Can you work these out from the model? Positions are in its coordinate system, mm. Give positions to 0.01 mm unless a question says otherwise; leave off trailing zeros. Order: outer loops, then holes, each group sorted by start corner. A loop starts at its lowest first (then second) coordinate and runs counter-clockwise, first axis right, second up. Notation, with made-up numbers: M -10.75,-29 L 42.25,-29 A19 cw 42.25,-25 Z; hole C 40.25,25.5 d2. An arc over 180 degrees is marked long. One line per question, with ' | ' between items. Start each with the question number.
1) If we section it at A-A, the plane y = 2.5: Please give me the cut outline in (x, z) (1 decimal).
2) I'm going to push flat-ended pins straight in: pin 1 Ø1.1 at (x, z) = (-29, 2) entering from +Y; pin 2 Ø8 at (x, z) = (-2, -164.5) entering from -Y. Where does each tip first touch, or does it pass through?
3) If we section it at B-B, the plane z = -77.5: Please give me the cut outline in (x, y).
4) Please list where these lines run through material, in increasing order: line 1 along Z through (x, y) = (-21, 2.55) (1 decimal); line 2 along X through (y, z) = (0.9, -141); line 3 along Z through (x, y) = (-38.5, 1.1) (1 decimal). Write a range as [from, to].
Autodesk Inventor part; units mm, degrees
ref_plane "YZ Plane" through (0, 0, 0) normal (1, 0, 0) x (0, 1, 0)
ref_plane "XZ Plane" through (0, 0, 0) normal (0, 1, 0) x (-1, 0, 0)
ref_plane "XY Plane" through (0, 0, 0) normal (0, 0, 1) x (1, 0, 0)
sketch "Sketch1" plane through (0, 0, 0) normal (0, 1, 0) x (-1, 0, 0)
  line L0 (0, 0) -> (50, 0)
  line L1 (50, 0) -> (50, -447.675)
  line L2 (50, -447.675) -> (0, -447.675)
  line L3 (0, -447.675) -> (0, 0)
  dimension "d0" = 50
  dimension "d1" = 447.675
extrude "Extrusion1" add sketch "Sketch1" along normal blind 4.7625
sketch "Sketch2" plane through (-50, 0, 0) normal (0, 0, 1) x (1, 0, 0)
  line L0 (1.1907, 3.5648) -> (1.1907, 1.1907)
  line L1 (50, 0) -> (0, 0)
  line L2 (50, 4.7625) -> (0, 4.7625)
  line L3 (1.1907, 1.1907) -> (48.8093, 1.1907)
  line L4 (1.1907, 3.5648) -> (48.8093, 3.5648)
  line L5 (48.8093, 3.5648) -> (48.8093, 1.1907)
  line L6 (50, 0) -> (50, 4.7625)
extrude "Extrusion2" add sketch "Sketch2" along normal blind 4.7625
sketch "Sketch3" plane through (0, 4.7625, 0) normal (0, 1, 0) x (1, 0, 0)
  line L0 (-50, 447.675) -> (-50, 0)
  line L1 (-50, 447.675) -> (-25, 447.675)
  line L2 (0, 447.675) -> (-50, 447.675)
  line L3 (-25, 447.675) -> (-25, 382.675)
  line L4 (-31, 382.675) -> (-19, 382.675)
  line L5 (-31, 382.675) -> (-31, 0)
  line L6 (-1.1907, 0) -> (-48.8093, 0)
  line L7 (-19, 382.675) -> (-19, 0)
  line L8 (-31, 0) -> (-19, 0)
  point P0 (0, 0)
  dimension "d11" = 25
extrude "Extrusion3" cut sketch "Sketch3" against normal blind 10
sketch "Sketch4" plane through (-50, 0, 4.7625) normal (0, 0, 1) x (1, 0, 0)
  line L0 (31, 3.5648) -> (31, 1.1907)
  line L1 (31, 1.1907) -> (31, 3.5648)
  line L2 (19, 3.5648) -> (31, 3.5648)
  line L3 (31, 3.5648) -> (19, 3.5648)
  line L4 (19, 3.5648) -> (19, 1.1907)
  line L5 (19, 1.1907) -> (31, 1.1907)
  point P0 (50, 0)
extrude "Extrusion4" cut sketch "Sketch4" against normal blind 10
sketch "Sketch5" plane through (0, 4.7625, 0) normal (0, 1, 0) x (1, 0, 0)
  point P0 (0, 0)
sketch "Sketch6" plane through (-31, 4.7625, -382.675) normal (0, 0, 1) x (1, 0, 0)
  line L0 (12, -4.7625) -> (0, -4.7625)
  line L1 (12, 0) -> (12, -4.7625)
  line L2 (0, 0) -> (12, 0)
  line L3 (0, 0) -> (0, -4.7625)
  point P0 (31, -4.7625)
extrude "Extrusion5" add sketch "Sketch6" along normal blind 158.838
sketch "Sketch8" plane through (-31, 4.7625, -223.837) normal (0, 0, 1) x (1, 0, 0)
  line L0 (3.6185, -4.7625) -> (3.6185, 0)
  line L1 (3.6185, 0) -> (8.3815, 0)
  line L2 (8.3815, 0) -> (8.3815, -4.7625)
  line L3 (3.6185, -4.7625) -> (8.3815, -4.7625)
  line L4 (0, -4.7625) -> (12, -4.7625)
  line L5 (-19, 0) -> (0, 0)
  line L6 (0, 0) -> (3.6185, 0)
  line L7 (12, 0) -> (0, 0)
  line L8 (3.6185, -4.7625) -> (0, -4.7625)
  line L9 (0, -4.7625) -> (0, 0)
  line L10 (0, -4.7625) -> (0, 0)
  line L11 (8.3815, 0) -> (12, 0)
  line L12 (12, -3.5718) -> (12, -4.7625)
  line L13 (12, -4.7625) -> (8.3815, -4.7625)
  line L14 (12, -4.7625) -> (12, 0)
  point P0 (31, -4.7625)
  dimension "d25" = 4.763
extrude "Extrusion6" add sketch "Sketch8" along normal blind 223.837 contours L4 L9 L6 L0 | L2 L7 L14 L12 L4
sketch "Sketch9" plane through (-19, 1.1907, 0) normal (-1, 0, 0) x (0, 0, 1)
  line L0 (0, 2.374) -> (0, 0)
  line L1 (4.7625, 0) -> (0, 0)
  line L2 (4.7625, 2.374) -> (4.7625, 0)
  line L3 (0, 2.374) -> (4.7625, 2.374)
  point P0 (0, -1.1907)
extrude "Extrusion7" add sketch "Sketch9" along normal blind 15
sketch "Sketch10" plane through (-22.6185, 3.5648, 0) normal (0, 0, -1) x (-1, 0, 0)
  line L0 (4.763, -2.374) -> (4.763, 0)
  line L1 (0, 0) -> (4.763, 0)
  line L2 (0, 0) -> (0, -2.374)
  line L3 (0, -2.374) -> (4.763, -2.374)
  point P0 (-22.6185, -3.5648)
extrude "Extrusion8" cut sketch "Sketch10" against normal blind 15
sketch "Sketch14" plane through (0, 4.7625, 0) normal (0, 1, 0) x (1, 0, 0)
  line L0 (0, 447.675) -> (-50, 447.675)
  line L1 (0, 0) -> (0, 447.675)
  line L2 (-50, 447.675) -> (-50, 0)
  line L3 (-27.3815, 223.837) -> (-27.3815, 0)
  line L4 (-22.6185, 223.837) -> (-22.6185, 0)
  line L5 (-5, 231.488) -> (-22.6185, 231.488)
  line L6 (-22.6185, 231.488) -> (-22.6185, 233.862)
  line L7 (-22.6185, 233.862) -> (-5, 233.862)
  line L8 (-5, 231.488) -> (-5, 233.862)
  line L9 (-27.3815, 223.837) -> (-22.6185, 223.837)
  line L10 (-45, 231.488) -> (-27.3815, 231.488)
  line L11 (-27.3815, 231.488) -> (-27.3815, 233.862)
  line L12 (-27.3815, 233.862) -> (-45, 233.862)
  line L13 (-45, 231.488) -> (-45, 233.862)
  dimension "d35" = 2.374
extrude "Extrusion9" cut sketch "Sketch14" against normal blind 10
sketch "Sketch17" plane through (0, 4.7625, 0) normal (0, 1, 0) x (1, 0, 0)
  line L0 (-50, 447.675) -> (-50, 0)
  line L1 (-50, 235.0565) -> (0, 235.0565)
  line L2 (0, 0) -> (0, 447.675)
  line L3 (-45, 231.488) -> (-45, 233.862)
  line L4 (-45, 236.2515) -> (-45, 238.6255)
  line L5 (-45, 238.6255) -> (-27.3815, 238.6255)
  line L6 (-45, 236.2515) -> (-27.3815, 236.2515)
  line L7 (-27.3815, 238.6255) -> (-27.3815, 236.2515)
  line L8 (-5, 236.2515) -> (-5, 238.6255)
  line L9 (-5, 238.6255) -> (-22.6185, 238.6255)
  line L10 (-5, 236.2515) -> (-22.6185, 236.2515)
  line L11 (-22.6185, 238.6255) -> (-22.6185, 236.2515)
  point P0 (-27.3815, 231.488)
  dimension "d43" = 2.374
extrude "Extrusion10" cut sketch "Sketch17" against normal blind 10
sketch "Sketch18" plane through (0, 4.7625, 0) normal (0, 1, 0) x (1, 0, 0)
  line L0 (-45, 233.862) -> (-45, 231.488)
  line L1 (-45, 233.862) -> (-45, 231.488)
  line L2 (-27.3815, 233.862) -> (-45, 233.862)
  line L3 (-45, 233.862) -> (-27.3815, 233.862)
  line L4 (-27.3815, 233.862) -> (-27.3815, 231.488)
  line L5 (-27.3815, 233.862) -> (-27.3815, 231.488)
  line L6 (-27.3815, 231.488) -> (-45, 231.488)
  line L7 (-22.6185, 231.488) -> (-5, 231.488)
  line L8 (-5, 231.488) -> (-22.6185, 231.488)
  line L9 (-22.6185, 231.488) -> (-22.6185, 233.862)
  line L10 (-22.6185, 233.862) -> (-5, 233.862)
  line L11 (-5, 231.488) -> (-5, 233.862)
  line L12 (-5, 233.862) -> (-5, 231.488)
  point P0 (0, 0)
extrude "Extrusion11" add sketch "Sketch18" against normal up to surface (4.7625 mm away)
sketch "Sketch19" plane through (0, 4.7625, 0) normal (0, 1, 0) x (1, 0, 0)
  line L0 (0, 0) -> (0, 447.675)
  line L1 (0, 0) -> (37.5, 0)
  line L2 (0, 447.675) -> (-50, 447.675)
  line L3 (0, 447.675) -> (37.5, 447.675)
  line L4 (37.5, 447.675) -> (37.5, 0)
  line L5 (0, 0) -> (0, 447.675)
  line L6 (-50, 0) -> (-50, 447.675)
  line L7 (-50, 0) -> (-87.5, 0)
  line L8 (-50, 447.675) -> (-87.5, 447.675)
  line L9 (-87.5, 447.675) -> (-87.5, 0)
  dimension "d48" = 37.5
  dimension "d49" = 37.5
extrude "Extrusion12" add sketch "Sketch19" against normal up to surface (4.7625 mm away)
sketch "Sketch20" plane through (-1.1907, 1.1907, 0) normal (0, 0, 1) x (1, 0, 0)
  line L0 (37.4997, 0) -> (0, 0)
  line L1 (0, 2.374) -> (0, 0)
  line L2 (0, 0) -> (0, 2.374)
  line L3 (0, 2.374) -> (0, 0)
  line L4 (0, 2.374) -> (37.4997, 2.374)
  line L5 (37.4997, 2.374) -> (37.4997, 0)
  line L6 (-26.1908, -1.1907) -> (-21.4278, -1.1907)
  line L7 (-21.4278, 3.5718) -> (-26.1908, 3.5718)
  line L8 (-85.1183, 0) -> (-47.6185, 0)
  line L9 (-47.6185, 2.374) -> (-47.6185, 0)
  line L10 (-47.6185, 2.374) -> (-85.1183, 2.374)
  line L11 (-85.1183, 2.374) -> (-85.1183, 0)
extrude "Extrusion13" add sketch "Sketch20" along normal up to surface (4.7625 mm away)
sketch "Sketch21" plane through (0, 4.7625, 0) normal (0, 1, 0) x (1, 0, 0)
  line L0 (-22.6185, 236.2515) -> (-5, 236.2515)
  line L1 (-22.6185, 236.2515) -> (9.8845, 236.2515)
  line L2 (-22.6185, 238.6255) -> (-22.6185, 236.2515)
  line L3 (9.8845, 238.6255) -> (9.8845, 236.2515)
  line L4 (-22.6185, 238.6255) -> (-22.6185, 236.2515)
  line L5 (-27.3815, 223.837) -> (-22.6185, 223.837)
  line L6 (-22.6185, 238.6255) -> (9.8845, 238.6255)
  line L7 (-27.3815, 236.2515) -> (-59.8845, 236.2515)
  line L8 (-27.3815, 238.6255) -> (-27.3815, 236.2515)
  line L9 (-59.8845, 238.6255) -> (-59.8845, 236.2515)
  line L10 (-27.3815, 238.6255) -> (-59.8845, 238.6255)
  point P0 (0, 0)
extrude "Extrusion14" cut sketch "Sketch21" against normal blind 10
properties part number "Sustainable Chair_V2 - Leg(A)_2_CPY" material "Foam Board - V3"
Results found:
1) outline: M -87.5,-447.7 L 37.5,-447.7 L 37.5,0 L 36.3,0 L 36.3,4.8 L -22.6,4.8 L -22.6,-223.8 L -27.4,-223.8 L -27.4,4.8 L -86.3,4.8 L -86.3,0 L -87.5,0 Z; hole M -59.9,-238.6 L -27.4,-238.6 L -27.4,-236.3 L -59.9,-236.3 Z; hole M -22.6,-238.6 L 9.9,-238.6 L 9.9,-236.3 L -22.6,-236.3 Z
2) pin 1: stops at y = 3.56 | pin 2: stops at y = 0
3) outline: M -87.5,0 L -27.38,0 L -27.38,4.76 L -87.5,4.76 Z; M -22.62,0 L 37.5,0 L 37.5,4.76 L -22.62,4.76 Z
4) line 1: z = [-447.7, -238.6], [-236.3, 4.8] | line 2: x = [-87.5, -27.38], [-22.62, 37.5] | line 3: z = [-447.7, -238.6], [-236.3, 0]
